Can you work these out from the model? Positions are in its coordinate system, mm. Face numbers are marked on the shaded views. A direction names the side the tool comes from. Coordinates: 2 decimals unless noted, no trailing zeros. Loops run counter-clockwise (first coordinate to the right, second up) from the corner with the lowest first, then second, coordinate; pieces in that order, holes last. Notation, with made-up numbers: M 77,-19.75 L 122,-19.75 A24 ccw 122,-4.75 Z; hole C 25.25,7 d3. An arc over 180 degrees is marked long. Answer as a JSON object with one key per item and string values. Group by question number.
Item 1: Suppose I cut it at D-D (x = 0). Write out the boundary of the cut face in (y, z), then the cut area to 3 significant figures.
Item 2: Suppose I cut it at C-C (x = 7). Write out the boundary of the cut face in (y, z), then the cut area to 3 significant figures.
Item 3: If I drill on line 1 (Z direction, x = 2, y = 89); line 2 (X direction, y = 33, z = 19.5); line 3 (X direction, y = 14.5, z = 16.5), over which ranges is the centre line in solid material (lowest first)?
Item 4: Suppose I cut it at B-B (y = 6). Write out the boundary of the cut face in (x, z), then the cut area to 3 significant figures.
Item 5: Which directions (+Z, -Z, +X, -X, +Y, -Y) give clear straight access to the entire face, cutting with the end or side of a thin tool? Please do the marked faces 4 and 5.
Item 6: We'd pull the mould along Y, two halves only. Please class the marked faces 1, 2 and 3: +Y half, -Y half, draft (parallel to the pull), parting line (faces both ways), or undercut.
Item 7: I'm going to push flat-ended pins straight in: pin 1 Ø10 at (y, z) = (106, 16) entering from +X; pin 2 Ø12 at (x, z) = (22.5, 40.5) entering from +Y; pin 3 Ø3 at (x, z) = (5.5, 10) entering from -Y. Where does each tip first touch, or does it pass through?
Item 8: Suppose I cut it at A-A (z = 10). Write out the boundary of the cut face in (x, y), then the cut area to 3 significant figures.
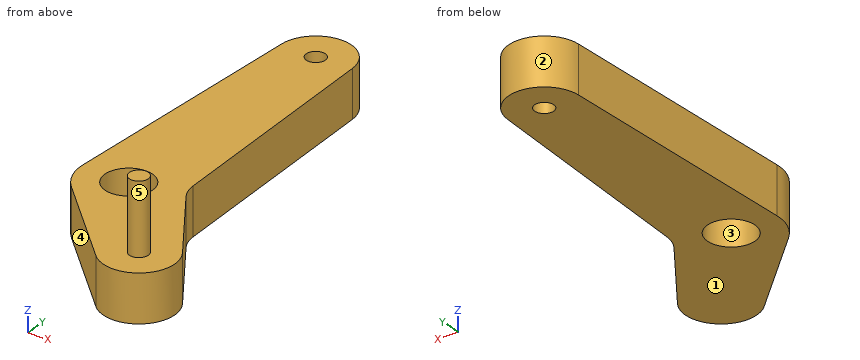
```python
from build123d import *

# Parameters (mm, degrees)
SKETCH_1_R      = 10
SKETCH_1_R_2    = 4
EXTRUDE_1_DEPTH = 20
SKETCH_3_R      = 4
EXTRUDE_2_DEPTH = 30


with BuildPart() as part:
    # 草图1 → 凸台-拉伸1 (new body)
    with BuildSketch(Plane.XY):
        with BuildLine():
            Line((-14.98449612, 110.681818182), (-19.97932816, 0.909090909))
            ThreePointArc((-19.97932816, 0.909090909), (-18.614490773, -7.314419545), (-14.01590192, -14.267252481))
            Line((-14.01590192, -14.267252481), (21.473440532, -49.131368307))
            ThreePointArc((21.473440532, -49.131368307), (41.580977064, -49.96020763), (44.416415431, -30.036345322))
            Line((44.416415431, -30.036345322), (22.085208252, 3.03263475))
            ThreePointArc((22.085208252, 3.03263475), (20.276358226, 6.712847666), (19.53176059, 10.745400192))
            Line((19.53176059, 10.745400192), (14.98449612, 110.681818182))
            ThreePointArc((14.98449612, 110.681818182), (0, 125), (-14.98449612, 110.681818182))
        make_face()
        Circle(SKETCH_1_R, mode=Mode.SUBTRACT)
        with Locations((0, 110)):
            Circle(SKETCH_1_R_2, mode=Mode.SUBTRACT)
    extrude(amount=EXTRUDE_1_DEPTH)

    # 草图3 → 凸台-拉伸2 (add)
    with BuildSketch(Plane.XY.offset(20)):
        with Locations(Location((31.985366972, -38.430928946, 0), (0, 0, 180))):
            Circle(SKETCH_3_R)
    extrude(amount=EXTRUDE_2_DEPTH)


solid = part.part
```
From the geometry:
{
 "1": {"outline": "M -28.04,0 L -10,0 L -10,20 L -28.04,20 Z; M 10,0 L 106,0 L 106,20 L 10,20 Z; M 114,0 L 125,0 L 125,20 L 114,20 Z", "area": "2,500 mm2"},
 "2": {"outline": "M -34.91,0 L -7.14,0 L -7.14,20 L -34.91,20 Z; M 7.14,0 L 123.27,0 L 123.27,20 L 7.14,20 Z", "area": "2,880 mm2"},
 "3": {"line 1": "0 to 20", "line 2": "-18.52 to 18.52", "line 3": "-19.36 to 19.36"},
 "4": {"outline": "M -19.75,0 L -8,0 L -8,20 L -19.75,20 Z; M 8,0 L 20.53,0 L 20.53,20 L 8,20 Z", "area": "486 mm2"},
 "5": {"face 4": "+Z, -Z, -X, -Y", "face 5": "+Z"},
 "6": {"face 1": "draft", "face 2": "+Y half", "face 3": "undercut"},
 "7": {"pin 1": "x = 15.43", "pin 2": "y = -36.47", "pin 3": "y = -34.91"},
 "8": {"outline": "M -19.98,0.91 A20 ccw -14.02,-14.27 L 21.47,-49.13 A15 ccw 44.42,-30.04 L 22.09,3.03 A15 cw 19.53,10.75 L 14.98,110.68 A15 ccw -14.98,110.68 Z; hole C 0,0 d20; hole C 0,110 d8", "area": "5,950 mm2"}
}
